Check sheet for the modelled part. Datum: model origin and axes. Units: mm. A direction names the side the tool comes from. Coordinates: 2 decimals unless noted, no trailing zeros. Loops run counter-clockwise (first coordinate to the right, second up) from the corner with the lowest first, then second, coordinate; pieces in that order, holes last. Notation, with made-up numbers: (80.25, -26.5) -> (137.25, -26.5) arc R7 ccw to (137.25, -19.5) -> close; hole circle Ø6 at (3.5, -28). An arc over 180 degrees is marked (long way). Use one line per item in the form item = value.
from build123d import *

# Parameters (mm, degrees)
SKETCH1_R               = 4.5
SKETCH1_R_2             = 1.25
BOSS_EXTRUDE1_DEPTH     = 8
SKETCH2_R               = 1.75
SKETCH2_R_2             = 1.25
CUT_EXTRUDE1_DEPTH      = 4
SKETCH4_W               = 12
SKETCH4_H               = 12
SKETCH4_W_2             = 6.5
SKETCH4_H_2             = 6.5
BOSS_EXTRUDE2_DEPTH     = 15
SKETCH5_W               = 15
SKETCH5_H               = 12
BOSS_EXTRUDE3_DEPTH     = 8
CUT_EXTRUDE2_DEPTH      = 24.769728648
CUT_EXTRUDE2_DEPTH_BACK = 24.769728648
SKETCH6_R               = 1.1
FILLET1_R               = 2
CUT_EXTRUDE3_START      = -1.5
SKETCH7_W               = 10
SKETCH7_H               = 15
SKETCH7_R               = 1.1
CUT_EXTRUDE3_DEPTH      = 1.5
CUT_EXTRUDE4_START      = -12
SKETCH7_2_W             = 10
SKETCH7_2_H             = 15
SKETCH7_2_R             = 1.1
CUT_EXTRUDE4_DEPTH      = 1.5
FILLET2_R               = 2
SKETCH1_2_R             = 4.5
SKETCH1_2_R_2           = 1.25
CUT_EXTRUDE5_DEPTH      = 8
BOSS_EXTRUDE5_OUTLINE_W = 6.5
BOSS_EXTRUDE5_OUTLINE_H = 6.5
BOSS_EXTRUDE5_OUTLINE_R = 1.75
BOSS_EXTRUDE5_DEPTH     = 3
SKETCH8_R               = 2.2
CUT_EXTRUDE6_DEPTH      = 14


with BuildPart() as part:
    # Sketch1 → Boss-Extrude1 (new body)
    with BuildSketch(Plane.XY):
        Circle(SKETCH1_R)
        Circle(SKETCH1_R_2, mode=Mode.SUBTRACT)
    extrude(amount=BOSS_EXTRUDE1_DEPTH)

    # Sketch2 → Cut-Extrude1 (cut)
    with BuildSketch(Plane(origin=(0, 0, 0), x_dir=(-1, 0, 0), z_dir=(0, 0, -1))):
        Circle(SKETCH2_R)
        Circle(SKETCH2_R_2, mode=Mode.SUBTRACT)
    extrude(amount=-CUT_EXTRUDE1_DEPTH, mode=Mode.SUBTRACT)

    # Sketch4 → Boss-Extrude2 (add)
    with BuildSketch(Plane(origin=(0, 0, 0), x_dir=(-1, 0, 0), z_dir=(0, 0, -1))):
        Rectangle(SKETCH4_W, SKETCH4_H)
        Rectangle(SKETCH4_W_2, SKETCH4_H_2, mode=Mode.SUBTRACT)
    extrude(amount=BOSS_EXTRUDE2_DEPTH)

    # Sketch5 → Boss-Extrude3 (add)
    with BuildSketch(Plane(origin=(6, 0, 0), x_dir=(0, 0, -1), z_dir=(1, 0, 0))):
        with Locations((7.5, 0)):
            Rectangle(SKETCH5_W, SKETCH5_H)
    extrude(amount=BOSS_EXTRUDE3_DEPTH)

    # Sketch6 → Cut-Extrude2 (cut, two sides: drawn at the far end of the back side and taken through both)
    with BuildSketch(Plane(origin=(0, 6, 0), x_dir=(1, 0, 0), z_dir=(0, 1, 0)).offset(-CUT_EXTRUDE2_DEPTH_BACK)):
        with Locations(Location((9, 11.25, 0), (0, 0, 270))):
            Circle(SKETCH6_R)
        with Locations(Location((9, 5, 0), (0, 0, 270))):
            Circle(SKETCH6_R)
    extrude(amount=CUT_EXTRUDE2_DEPTH + CUT_EXTRUDE2_DEPTH_BACK, mode=Mode.SUBTRACT)

    # Fillet1
    fillet1_edges = [part.edges().sort_by_distance(p)[0] for p in [
        (-6, -6, -7.5),
        (-6, 6, -7.5),
    ]]
    fillet(fillet1_edges, radius=FILLET1_R)

    # Sketch7 → Cut-Extrude3 (cut)
    with BuildSketch(Plane.XZ.offset(6).offset(CUT_EXTRUDE3_START)):
        with Locations((9, -7.5)):
            Rectangle(SKETCH7_W, SKETCH7_H)
        with Locations(Location((9, -5, 0), (0, 0, 270))):
            Circle(SKETCH7_R, mode=Mode.SUBTRACT)
    extrude(amount=CUT_EXTRUDE3_DEPTH, mode=Mode.SUBTRACT)

    # Sketch7<2> → Cut-Extrude4 (cut)
    with BuildSketch(Plane.XZ.offset(6).offset(CUT_EXTRUDE4_START)):
        with Locations((9, -7.5)):
            Rectangle(SKETCH7_2_W, SKETCH7_2_H)
        with Locations(Location((9, -5, 0), (0, 0, 270))):
            Circle(SKETCH7_2_R, mode=Mode.SUBTRACT)
    extrude(amount=CUT_EXTRUDE4_DEPTH, mode=Mode.SUBTRACT)

    # Fillet2
    # the kernel refuses this fillet: 2 mm, written as the material it adds along each edge
    with BuildSketch(Plane(origin=(4, 4.5, 0), x_dir=(1, 0, 0), z_dir=(0, 0, -1))) as fillet2_piece_1:
        with BuildLine():
            CenterArc((1.936491673, -2), FILLET2_R, 90, 75.522487814)
            Line((0, -1.5), (0, 0))
            Line((0, 0), (1.936491673, 0))
        make_face()
    extrude(amount=15)
    with BuildSketch(Plane(origin=(4, -4.5, 0), x_dir=(0, -1, 0), z_dir=(0, 0, -1))) as fillet2_piece_2:
        with BuildLine():
            CenterArc((2, -1.936491673), FILLET2_R, 104.477512186, 75.522487814)
            Line((0, -1.936491673), (0, 0))
            Line((0, 0), (1.5, 0))
        make_face()
    extrude(amount=15)
    # the kernel refuses this fillet: 2 mm, written as the material it takes off along each edge
    with BuildSketch(Plane(origin=(14, -4.5, -20), x_dir=(0, 1, 0), z_dir=(0, 0, 1)), Plane(origin=(14, 4.5, -20), x_dir=(-1, 0, 0), z_dir=(0, 0, 1))) as fillet2_2_piece_1:
        with BuildLine():
            CenterArc((FILLET2_R, FILLET2_R), FILLET2_R, 180, 90)
            Line((0, FILLET2_R), (0, 0))
            Line((0, 0), (FILLET2_R, 0))
        make_face()
    extrude(amount=25, mode=Mode.SUBTRACT)

    # Sketch1<2> → Cut-Extrude5 (cut)
    with BuildSketch(Plane.XY):
        Circle(SKETCH1_2_R)
        Circle(SKETCH1_2_R_2, mode=Mode.SUBTRACT)
    extrude(amount=CUT_EXTRUDE5_DEPTH, mode=Mode.SUBTRACT)

    # Boss-Extrude5: read off the stored shape, not the designer's step
    # Boss-Extrude5 outline → Boss-Extrude5 (add)
    with BuildSketch(Plane(origin=(0, 0, 0), x_dir=(-1, 0, 0), z_dir=(0, 0, -1))):
        Rectangle(BOSS_EXTRUDE5_OUTLINE_W, BOSS_EXTRUDE5_OUTLINE_H)
        Circle(BOSS_EXTRUDE5_OUTLINE_R, mode=Mode.SUBTRACT)
    extrude(amount=BOSS_EXTRUDE5_DEPTH)

    # Sketch8 → Cut-Extrude6 (cut)
    with BuildSketch(Plane.XZ.offset(6)):
        with Locations(Location((0, -7.5, 0), (0, 0, 270))):
            Circle(SKETCH8_R)
    extrude(amount=-CUT_EXTRUDE6_DEPTH, mode=Mode.SUBTRACT)


solid = part.part
(1) Section check C-C, the plane x = 9. Record the boundary of the cut face in (y, z).
Established:
outline = (-4.5, -15) -> (4.5, -15) -> (4.5, -12.35) -> (-4.5, -12.35) -> close; (-4.5, -10.15) -> (4.5, -10.15) -> (4.5, -6.1) -> (-4.5, -6.1) -> close; (-4.5, -3.9) -> (4.5, -3.9) -> (4.5, 0) -> (-4.5, 0) -> close
(2) Mould release check, pull along Y, two halves, no side actions. Record for faces 1 (the flat face through (9, 4.5, -7)), 2 (the flat face through (-3.25, 0, -9)), 3 (the flat face through (4, 0, -15)), 4 (the cylindrical face through (4.7, -4.93, -7.4)): +Y half, -Y half, draft (parallel to the pull), parting line (faces both ways), or undercut.
Established:
face_1 = +Y half
face_2 = undercut
face_3 = draft
face_4 = -Y half
(3) Section check A-A, the plane y = 0. Record the boundary of the cut face in (x, z).
Established:
outline = (-6, -15) -> (-3.25, -15) -> (-3.25, -3) -> (-1.75, -3) -> (-1.75, 0) -> (-6, 0) -> close; (1.75, -3) -> (3.25, -3) -> (3.25, -15) -> (14, -15) -> (14, 0) -> (1.75, 0) -> close; hole circle Ø2.2 at (9, -11.25); hole circle Ø2.2 at (9, -5)
(4) Section check D-D, the plane x = 0.25. Record the boundary of the cut face in (y, z), plus the area to 3 significant figures.
Established:
outline = (-6, -15) -> (-3.25, -15) -> (-3.25, -9.69) -> (-6, -9.69) -> close; (-6, -5.31) -> (-3.25, -5.31) -> (-3.25, -3) -> (-1.73, -3) -> (-1.73, 0) -> (-6, 0) -> close; (1.73, -3) -> (3.25, -3) -> (3.25, -5.31) -> (6, -5.31) -> (6, 0) -> (1.73, 0) -> close; (3.25, -15) -> (6, -15) -> (6, -9.69) -> (3.25, -9.69) -> close
area = 67.6 mm²
(5) Tool access check on faces 5 (the flat face through (2, 6, -6)), 6 (the flat face through (0, -3.25, -10)). Record the directions out of +Z, -Z, +X, -X, +Y, -Y that give a thin tool (end or side, any length) a straight path to the whole face; none if there is none.
Established:
face_5 = +Z, -Z, +X, -X, +Y
face_6 = -Z
(6) Scan lines: line 1 along X through (y, z) = (-1, -5); line 2 along Z through (x, y) = (9.5, -3.5); line 3 along Z through (x, y) = (8, 1.75). Record each from-to range of solid material in increasing order.
Established:
line_1 = -6 to -3.25, 3.25 to 7.9, 10.1 to 14
line_2 = -15 to -12.23, -10.27 to -5.98, -4.02 to 0
line_3 = -15 to -11.71, -10.79 to -5.46, -4.54 to 0
(7) Go/stop test with flat-tipped pins: P1, Ø3, axis at x = 11.5, z = -2, coming from the -Y side; P2, Ø6.5, axis at x = 9, z = -9.5, coming from the +Y side; P3, Ø2, axis at x = 9, z = -5, coming from the +Y side. Record where each tip stops, or that it passes through.
Established:
P1 = -4.5
P2 = 4.51
P3 = through
(8) Section check B-B, the plane z = -5. Record the boundary of the cut face in (x, y).
Established:
outline = (-6, -4) arc R2 ccw to (-4, -6) -> (4, -6) arc R2 cw to (5.94, -4.5) -> (7.9, -4.5) -> (7.9, 4.5) -> (5.94, 4.5) arc R2 cw to (4, 6) -> (-4, 6) arc R2 ccw to (-6, 4) -> close; (10.1, -4.5) -> (12, -4.5) arc R2 ccw to (14, -2.5) -> (14, 2.5) arc R2 ccw to (12, 4.5) -> (10.1, 4.5) -> close; hole (-3.25, -3.25) -> (3.25, -3.25) -> (3.25, 3.25) -> (-3.25, 3.25) -> close
